The model under review builds one solid part; all positions refer to its coordinate system, in mm. Give positions to 0.01 mm unless a question says otherwise; leave off trailing zeros. Return JSON: item names as keys, results as strings. Group by question number.
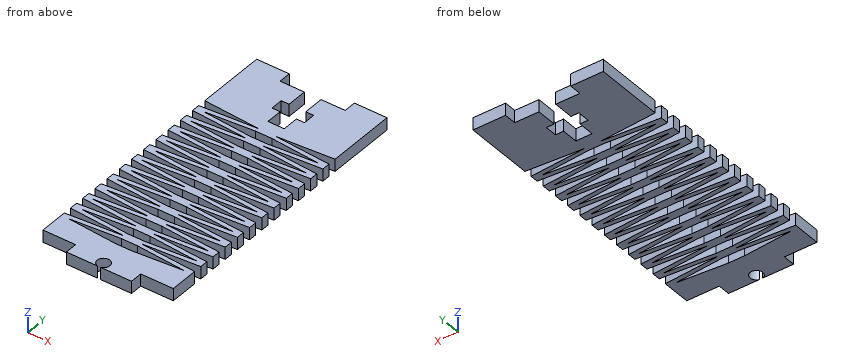
```python
from build123d import *

# Parameters (mm, degrees)
EXTRUDE_1_DEPTH = 3


with BuildPart() as part:
    # 草图2 → 凸台-拉伸1 (new body)
    with BuildSketch(Plane.XY):
        with BuildLine():
            Line((2.047890023, 48.855305477), (8, 48.855305477))
            Line((8, 48.855305477), (8, 51.855305477))
            Line((8, 51.855305477), (16, 51.855305477))
            Line((16, 51.855305477), (16, 34.855305477))
            Line((16, 34.855305477), (2, 33.855305477))
            Line((2, 33.855305477), (16, 32.855305477))
            Line((16, 32.855305477), (16, 30.855305477))
            Line((16, 30.855305477), (2, 29.855305477))
            Line((2, 29.855305477), (16, 28.855305477))
            Line((16, 28.855305477), (16, 26.855305477))
            Line((16, 26.855305477), (2, 25.855305477))
            Line((2, 25.855305477), (16, 24.855305477))
            Line((16, 24.855305477), (16, 22.855305477))
            Line((16, 22.855305477), (2, 21.855305477))
            Line((2, 21.855305477), (16, 20.855305477))
            Line((16, 20.855305477), (16, 18.855305477))
            Line((16, 18.855305477), (2, 17.855305477))
            Line((2, 17.855305477), (16, 16.855305477))
            Line((16, 16.855305477), (16, 14.855305477))
            Line((16, 14.855305477), (2, 13.855305477))
            Line((2, 13.855305477), (16, 12.855305477))
            Line((16, 12.855305477), (16, 10.855305477))
            Line((16, 10.855305477), (2, 9.855305477))
            Line((2, 9.855305477), (16, 8.855305477))
            Line((16, 8.855305477), (16, 6.855305477))
            Line((16, 6.855305477), (2, 5.855305477))
            Line((2, 5.855305477), (16, 4.855305477))
            Line((16, 4.855305477), (16, 2.855305477))
            Line((16, 2.855305477), (2, 1.855305477))
            Line((2, 1.855305477), (16, 0.855305477))
            Line((16, 0.855305477), (16, -1.144694523))
            Line((16, -1.144694523), (2, -2.144694523))
            Line((2, -2.144694523), (16, -3.144694523))
            Line((16, -3.144694523), (16, -5.144694523))
            Line((16, -5.144694523), (2, -6.144694523))
            Line((2, -6.144694523), (16, -7.144694523))
            Line((16, -7.144694523), (16, -9.144694523))
            Line((16, -9.144694523), (2, -10.144694523))
            Line((2, -10.144694523), (16, -11.144694523))
            Line((16, -11.144694523), (16, -18.144694523))
            Line((16, -18.144694523), (8, -18.144694523))
            Line((8, -18.144694523), (8, -21.144694523))
            Line((8, -21.144694523), (0.390512484, -21.144694523))
            ThreePointArc((0.390512484, -21.144694523), (0, -18.094694523), (-0.390512484, -21.144694523))
            Line((-0.390512484, -21.144694523), (-8, -21.144694523))
            Line((-8, -21.144694523), (-8, -18.144694523))
            Line((-8, -18.144694523), (-16, -18.144694523))
            Line((-16, -18.144694523), (-16, -11.144694523))
            Line((-16, -11.144694523), (-2, -10.144694523))
            Line((-2, -10.144694523), (-16, -9.144694523))
            Line((-16, -9.144694523), (-16, -7.144694523))
            Line((-16, -7.144694523), (-2, -6.144694523))
            Line((-2, -6.144694523), (-16, -5.144694523))
            Line((-16, -5.144694523), (-16, -3.144694523))
            Line((-16, -3.144694523), (-2, -2.144694523))
            Line((-2, -2.144694523), (-16, -1.144694523))
            Line((-16, -1.144694523), (-16, 0.855305477))
            Line((-16, 0.855305477), (-2, 1.855305477))
            Line((-2, 1.855305477), (-16, 2.855305477))
            Line((-16, 2.855305477), (-16, 4.855305477))
            Line((-16, 4.855305477), (-2, 5.855305477))
            Line((-2, 5.855305477), (-16, 6.855305477))
            Line((-16, 6.855305477), (-16, 8.855305477))
            Line((-16, 8.855305477), (-2, 9.855305477))
            Line((-2, 9.855305477), (-16, 10.855305477))
            Line((-16, 10.855305477), (-16, 12.855305477))
            Line((-16, 12.855305477), (-2, 13.855305477))
            Line((-2, 13.855305477), (-16, 14.855305477))
            Line((-16, 14.855305477), (-16, 16.855305477))
            Line((-16, 16.855305477), (-2, 17.855305477))
            Line((-2, 17.855305477), (-16, 18.855305477))
            Line((-16, 18.855305477), (-16, 20.855305477))
            Line((-16, 20.855305477), (-2, 21.855305477))
            Line((-2, 21.855305477), (-16, 22.855305477))
            Line((-16, 22.855305477), (-16, 24.855305477))
            Line((-16, 24.855305477), (-2, 25.855305477))
            Line((-2, 25.855305477), (-16, 26.855305477))
            Line((-16, 26.855305477), (-16, 28.855305477))
            Line((-16, 28.855305477), (-2, 29.855305477))
            Line((-2, 29.855305477), (-16, 30.855305477))
            Line((-16, 30.855305477), (-16, 32.855305477))
            Line((-16, 32.855305477), (-2, 33.855305477))
            Line((-2, 33.855305477), (-16, 34.855305477))
            Line((-16, 34.855305477), (-16, 51.855305477))
            Line((-16, 51.855305477), (-8, 51.855305477))
            Line((-8, 51.855305477), (-8, 48.855305477))
            Line((-8, 48.855305477), (-2.047890023, 48.855305477))
            Line((-2.047890023, 48.855305477), (-2.047890023, 43.855305477))
            Line((-2.047890023, 43.855305477), (-4, 43.855305477))
            Line((-4, 43.855305477), (-4, 40.855305477))
            Line((-4, 40.855305477), (-2, 40.855305477))
            Line((-2, 40.855305477), (-2, 36.855305477))
            Line((-2, 36.855305477), (2, 36.855305477))
            Line((2, 36.855305477), (2, 40.855305477))
            Line((2, 40.855305477), (4, 40.855305477))
            Line((4, 40.855305477), (4, 43.855305477))
            Line((4, 43.855305477), (2.047890023, 43.855305477))
            Line((2.047890023, 43.855305477), (2.047890023, 48.855305477))
        make_face()
        Polygon((-14.217878812, -12.144694523), (-2, -13.144694523), (2, -13.144694523), (14.217878812, -12.144694523), (2, -11.144694523), (-2, -11.144694523), align=None, mode=Mode.SUBTRACT)
        Polygon((2, 32.855305477), (14.217878812, 31.855305477), (2, 30.855305477), (-2, 30.855305477), (-14.217878812, 31.855305477), (-2, 32.855305477), align=None, mode=Mode.SUBTRACT)
        Polygon((2, 28.855305477), (14.217878812, 27.855305477), (2, 26.855305477), (-2, 26.855305477), (-14.217878812, 27.855305477), (-2, 28.855305477), align=None, mode=Mode.SUBTRACT)
        Polygon((2, 24.855305477), (14.217878812, 23.855305477), (2, 22.855305477), (-2, 22.855305477), (-14.217878812, 23.855305477), (-2, 24.855305477), align=None, mode=Mode.SUBTRACT)
        Polygon((2, 20.855305477), (14.217878812, 19.855305477), (2, 18.855305477), (-2, 18.855305477), (-14.217878812, 19.855305477), (-2, 20.855305477), align=None, mode=Mode.SUBTRACT)
        Polygon((2, 16.855305477), (14.217878812, 15.855305477), (2, 14.855305477), (-2, 14.855305477), (-14.217878812, 15.855305477), (-2, 16.855305477), align=None, mode=Mode.SUBTRACT)
        Polygon((2, 12.855305477), (14.217878812, 11.855305477), (2, 10.855305477), (-2, 10.855305477), (-14.217878812, 11.855305477), (-2, 12.855305477), align=None, mode=Mode.SUBTRACT)
        Polygon((2, 8.855305477), (14.217878812, 7.855305477), (2, 6.855305477), (-2, 6.855305477), (-14.217878812, 7.855305477), (-2, 8.855305477), align=None, mode=Mode.SUBTRACT)
        Polygon((2, 4.855305477), (14.217878812, 3.855305477), (2, 2.855305477), (-2, 2.855305477), (-14.217878812, 3.855305477), (-2, 4.855305477), align=None, mode=Mode.SUBTRACT)
        Polygon((2, 0.855305477), (14.217878812, -0.144694523), (2, -1.144694523), (-2, -1.144694523), (-14.217878812, -0.144694523), (-2, 0.855305477), align=None, mode=Mode.SUBTRACT)
        Polygon((2, -3.144694523), (14.217878812, -4.144694523), (2, -5.144694523), (-2, -5.144694523), (-14.217878812, -4.144694523), (-2, -3.144694523), align=None, mode=Mode.SUBTRACT)
        Polygon((2, -7.144694523), (14.217878812, -8.144694523), (2, -9.144694523), (-2, -9.144694523), (-14.217878812, -8.144694523), (-2, -7.144694523), align=None, mode=Mode.SUBTRACT)
    extrude(amount=EXTRUDE_1_DEPTH)


solid = part.part
```
1) To check wall thickness, follow line 1 (X direction, y = 44.5, z = 2.1). State the ranges of the line that lie inside material, in increasing order.
2) For pin 1 Ø1.5 at (x, z) = (0.5, 2) entering from +Y; pin 2 Ø1 at (x, z) = (3.5, 2) entering from +Y, all flat-tipped, find the tip position at first contact; note any pin that passes through.
3) We need section A-A, the plane x = -9. Count the separate pieces of the cut face and the enclosed holes in it, plus the area to 3 significant figures.
Findings:
{
 "1": {"line 1": "x = -16 to -2.05, 2.05 to 16"},
 "2": {"pin 1": "stops at y = 36.86", "pin 2": "stops at y = 48.86"},
 "3": {"separate pieces": "25", "enclosed holes": "0", "area": "143 mm^2"}
}
